from build123d import *


with BuildPart() as part:
    # 草图1 → 旋转1 (revolve)
    with BuildSketch(Plane(origin=(0, 0, 0), x_dir=(1, 0, 0), z_dir=(0, 1, 0))):
        with BuildLine():
            Line((0, 0), (0, -8.5))
            ThreePointArc((0, -8.5), (0.146446609, -8.853553391), (0.5, -9))
            Line((0.5, -9), (5.5, -9))
            ThreePointArc((5.5, -9), (5.853553391, -8.853553391), (6, -8.5))
            Line((6, -8.5), (6, -4))
            Line((6, -4), (8, -4))
            Line((8, -4), (8, -3))
            Line((8, -3), (16, -3))
            Line((16, -3), (16, 0))
            Line((16, 0), (0, 0))
        make_face()
    revolve(axis=Axis((16, 0, 0), (-1, 0, 0)))


solid = part.part
Input: part model. Units: mm. Frame: model coordinates. A direction names the side the tool comes from. Coordinates: 2 decimals unless noted, no trailing zeros. Order: outer loops, then holes, each group sorted by start corner. A loop starts at its lowest first (then second) coordinate and runs counter-clockwise, first axis right, second up. Notation, with made-up numbers: M 4,45.5 L 33,45.5 A8 ccw 33,55.5 Z; hole C -35.5,74.5 d5. An arc over 180 degrees is marked long. Answer in a Markdown table with one row per item.
(1) Access query for faces 1 (the flat face through (16, 0, 0)), 2 (the cylindrical face through (7.014, -3.905, -0.867)). Directions: +Z, -Z, +X, -X, +Y, -Y. A direction counts if a zero-diameter tool reaches every point of the face in a straight line with its end or side. Return the directions, or none.
Numbers:
| item | result |
|---|---|
| face 1 | +Z, -Z, +X, +Y, -Y |
| face 2 | +X |
(2) Section query A-A, the plane z = 0. Output: boundary loops of the cut face in (x, y).
Numbers:
| item | result |
|---|---|
| outline | M 0,-8.5 A0.5 ccw 0.5,-9 L 5.5,-9 A0.5 ccw 6,-8.5 L 6,-4 L 8,-4 L 8,-3 L 16,-3 L 16,3 L 8,3 L 8,4 L 6,4 L 6,8.5 A0.5 ccw 5.5,9 L 0.5,9 A0.5 ccw 0,8.5 Z |
(3) Material intervals for line 1 (X direction, y = -4.25, z = -4.5); line 2 (Y direction, x = 3.5, z = 0.25); line 3 (Z direction, x = 10.5, y = 1.75), sorted ascending. Write a range as [from, to].
Numbers:
| item | result |
|---|---|
| line 1 | x = [0, 6] |
| line 2 | y = [-9, 9] |
| line 3 | z = [-2.44, 2.44] |
(4) Section query D-D, the plane x = 7.5. Output: boundary loops of the cut face in (y, z).
Numbers:
| item | result |
|---|---|
| outline | C 0,0 d8 |
(5) Section query C-C, the plane x = 12.75. Output: boundary loops of the cut face in (y, z), plus the area to 3 significant figures.
Numbers:
| item | result |
|---|---|
| outline | C 0,0 d6 |
| area | 28.3 mm^2 |
(6) Contact query for flat-ended pins moving along their axis: pin 1 Ø5 at (x, z) = (7.5, -6.5) entering from +Y; pin 2 Ø5 at (y, z) = (-6.5, -2.5) entering from +X; pin 3 Ø6 at (x, y) = (12.5, 4.5) entering from -Z. Output: stop coordinate, or through.
Numbers:
| item | result |
|---|---|
| pin 1 | stops at y = 7.59 |
| pin 2 | stops at x = 6 |
| pin 3 | stops at z = -2.6 |
